from build123d import *

# Parameters (mm, degrees)
SKETCH1_W            = 636.25984
SKETCH1_H            = 172.09262
BOSS_EXTRUDE1_DEPTH  = 3.175
SKETCH2_W            = 3.175
SKETCH2_H            = 3.175
CUT_EXTRUDE1_DEPTH   = 94.36608
SKETCH3_W            = 3.175
SKETCH3_H            = 3.175
CUT_EXTRUDE5_DEPTH   = 70.49262
SKETCH4_W            = 636.25984
SKETCH4_H            = 24.39416
CUT_EXTRUDE6_DEPTH   = 660.130134708
SKETCH6_W            = 636.25984
SKETCH6_H            = 24.39416
BOSS_EXTRUDE2_DEPTH  = 3.175
SKETCH7_W            = 254
SKETCH7_H            = 3.175
BOSS_EXTRUDE3_DEPTH  = 6.35
SKETCH8_R            = 2.25
CUT_EXTRUDE7_DEPTH   = 661.816489847
M4_CLEARANCE_HOLE1_D = 4.8


with BuildPart() as part:
    # Sketch1 → Boss-Extrude1 (new body)
    with BuildSketch(Plane(origin=(0, 0, 0), x_dir=(1, 0, 0), z_dir=(0, 1, 0))):
        with Locations((318.12992, 86.04631)):
            Rectangle(SKETCH1_W, SKETCH1_H)
    extrude(amount=BOSS_EXTRUDE1_DEPTH)

    # Sketch2 → Cut-Extrude1 (cut)
    with BuildSketch(Plane(origin=(0, 0, -172.09262), x_dir=(-1, 0, 0), z_dir=(0, 0, -1))):
        with Locations((-318.12992, 1.5875)):
            Rectangle(SKETCH2_W, SKETCH2_H)
    extrude(amount=-CUT_EXTRUDE1_DEPTH, mode=Mode.SUBTRACT)

    # Sketch3 → Cut-Extrude5 (cut)
    with BuildSketch(Plane.XY.offset(-172.09262)):
        with Locations((1.5875, 1.5875)):
            Rectangle(SKETCH3_W, SKETCH3_H)
        with Locations((634.67234, 1.5875)):
            Rectangle(SKETCH3_W, SKETCH3_H)
    extrude(amount=CUT_EXTRUDE5_DEPTH, mode=Mode.SUBTRACT)

    # Sketch4 → Cut-Extrude6 (cut, through all)
    with BuildSketch(Plane(origin=(0, 3.175, 0), x_dir=(1, 0, 0), z_dir=(0, 1, 0))):
        with Locations((318.12992, 12.19708)):
            Rectangle(SKETCH4_W, SKETCH4_H)
    extrude(amount=-CUT_EXTRUDE6_DEPTH, mode=Mode.SUBTRACT)

    # Sketch6 → Boss-Extrude2 (add, through all)
    with BuildSketch(Plane(origin=(0, 3.175, 0), x_dir=(1, 0, 0), z_dir=(0, 1, 0))):
        with Locations((318.12992, 12.19708)):
            Rectangle(SKETCH6_W, SKETCH6_H)
    extrude(amount=-BOSS_EXTRUDE2_DEPTH)

    # Sketch7 → Boss-Extrude3 (add)
    with BuildSketch(Plane(origin=(0, 0, -172.09262), x_dir=(-1, 0, 0), z_dir=(0, 0, -1))):
        with Locations((-476.40113, 1.5875)):
            Rectangle(SKETCH7_W, SKETCH7_H)
        with Locations((-159.85871, 1.5875)):
            Rectangle(SKETCH7_W, SKETCH7_H)
    extrude(amount=BOSS_EXTRUDE3_DEPTH)

    # Sketch8 → Cut-Extrude7 (cut, through all)
    with BuildSketch(Plane(origin=(0, 3.175, 0), x_dir=(1, 0, 0), z_dir=(0, 1, 0))):
        with Locations(Location((26.107106781, 10.16, 0), (0, 0, 270))):
            Circle(SKETCH8_R)
        with Locations(Location((172.118513391, 10.16, 0), (0, 0, 270))):
            Circle(SKETCH8_R)
        with Locations(Location((318.12992, 10.16, 0), (0, 0, 270))):
            Circle(SKETCH8_R)
        with Locations(Location((464.141326609, 10.16, 0), (0, 0, 270))):
            Circle(SKETCH8_R)
        with Locations(Location((610.152733219, 10.16, 0), (0, 0, 270))):
            Circle(SKETCH8_R)
    extrude(amount=-CUT_EXTRUDE7_DEPTH, mode=Mode.SUBTRACT)

    # M4 Clearance Hole1 (through all)
    with Locations(Plane(origin=(0, 3.175, 0), x_dir=(1, 0, 0), z_dir=(0, 1, 0))):
        with Locations((21.682533496, 18.397319949), (122.433944248, 18.397319949), (159.85871, 18.397319949), (197.283475752, 18.397319949), (298.034886505, 18.397319949), (338.224953495, 18.397319949), (438.976364248, 18.397319949), (476.40113, 18.397319949), (513.825895752, 18.397319949), (614.577306504, 18.397319949)):
            Hole(M4_CLEARANCE_HOLE1_D / 2)


solid = part.part
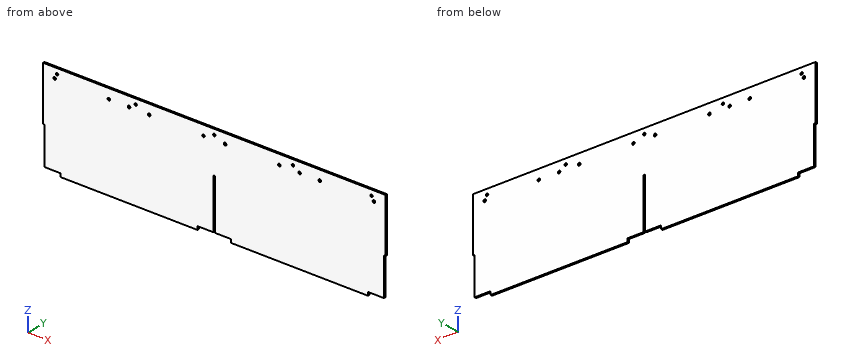
Can you work these out from the model? Positions are in its coordinate system, mm. Give positions to 0.01 mm unless a question says otherwise; leave off trailing zeros. Answer as a JSON object with one key per item and string values.
Q1. Imagine slicing it at A-A on y = 1.4. Give the number of separate pieces and of enclosed holes in the cut face, plus the area to 3 significant figures.
Geometry says:
{"separate pieces": "1", "enclosed holes": "15", "area": "112,000 mm²"}
Q2. Will these pins go through, and if not, where does the flat tip stop? P1, Ø1.6, axis at y = 1, z = -174.5, coming from the +X side; P2, Ø1, axis at y = 2, z = -118, coming from the -X side (3 decimals).
Geometry says:
{"P1": "x = 603.4", "P2": "x = 3.175"}
Q3. If I drill on L1, parallel to X at y = 2.3, z = -10.16; L2, parallel to X at y = 0.6, z = -138 (3 decimals); L3, parallel to Z at x = 198, y = 0.75, over which ranges is the centre line in solid material (lowest first)?
Geometry says:
{"L1": "0 to 23.86, 28.36 to 169.87, 174.37 to 315.88, 320.38 to 461.89, 466.39 to 607.9, 612.4 to 636.26", "L2": "3.175 to 316.542, 319.717 to 633.085", "L3": "-178.44 to -20.69, -16.11 to 0"}
